Autodesk Inventor part; units mm, degrees
ref_plane "YZ Plane" through (0, 0, 0) normal (1, 0, 0) x (0, 1, 0)
sketch "Sketch1" plane through (0, 0, 0) normal (0, 0, 1) x (1, 0, 0)
  line L0 (0, 0) -> (1.778, 0)
  line L1 (1.778, 0) -> (1.778, 5.08)
  line L2 (1.778, 5.08) -> (0, 5.08)
  line L3 (0, 5.08) -> (0, 0)
  line L4 (1.778, 0) -> (11.049, 0)
  line L5 (11.049, 0) -> (11.049, 3.683)
  line L6 (11.049, 3.683) -> (1.778, 3.683)
  line L7 (1.778, 3.683) -> (1.778, 0)
  line L8 (8.509, 3.683) -> (6.985, 3.81)
  line L9 (6.985, 3.81) -> (6.985, 3.683)
  line L10 (6.985, 3.683) -> (5.461, 3.81)
  line L11 (5.461, 3.81) -> (5.461, 3.683)
  line L12 (5.461, 3.683) -> (3.937, 3.81)
  line L13 (3.937, 3.81) -> (3.937, 3.683)
  line L14 (0, 0) -> (0, 3.1252)
  line L15 (0, 3.81) -> (0.889, 3.81) construction
  line L16 (0, 3.81) -> (0, 0)
  arc A0 (0, 3.81) -> (-9.906, 3.556) centre (0, -189.484) ccw
  line L17 (-9.906, 3.556) -> (-9.906, 3.81)
  line L18 (-9.906, 3.81) -> (-11.176, 3.81)
  line L19 (-11.176, 3.81) -> (-11.176, 0)
  line L20 (-11.176, 0) -> (0, 0)
  dimension "d0" = 1.778
  dimension "d1" = 10.16
  dimension "d2" = 9.271
  dimension "d3" = 7.366
  dimension "d4" = 7.62
  dimension "d5" = 2.54
  dimension "d6" = 1.524
  dimension "d7" = 7.62
  dimension "d8" = 7.62
  dimension "d9" = 11.176
  dimension "d10" = 7.112
  dimension "d11" = 1.27
revolve "Revolution1" add sketch "Sketch1" angle 360 about axis through (-11.176, 0, 0) along (1, 0, 0)
sketch "Sketch2" plane through (0, 0, 0) normal (0, 0, 1) x (1, 0, 0)
  line L0 (-11.176, 0.508) -> (-6.096, 0.508)
  line L1 (-6.096, 0.508) -> (-6.096, -0.508)
  line L2 (-6.096, -0.508) -> (-11.176, -0.508)
  line L3 (-11.176, -0.508) -> (-11.176, 0.508)
  line L4 (-11.176, -3.81) -> (-11.176, 3.81) construction
  point P0 (0, 0)
  point P1 (-11.176, 0)
  dimension "d13" = 1.016
  dimension "d14" = 5.08
extrude "Extrusion1" cut sketch "Sketch2" along normal through all both and the other way through all
hole "Hole1" at (-11.176, 0, 0) direction (1, 0, 0) diameter 4.7625 depth 11.1125 counterbore diameter 6.35 counterbore depth 6.35
hole "Hole2" at (11.049, 0, 0) direction (-1, 0, 0) diameter 4.7625 depth 9.525 counterbore diameter 6.35 counterbore depth 1.27
sketch "Sketch3" plane through (1.778, 0, 0) normal (1, 0, 0) x (0, 0, -1)
  circle A0 centre (0, 0) radius 5.08
  circle A1 centre (0, 0) radius 5.08
  circle A2 centre (0, 0) radius 3.683
  circle A3 centre (0, 0) radius 3.81
  circle A4 centre (0, 0) radius 3.81
  circle A5 centre (0, 0) radius 3.81
  circle A6 centre (0, 0) radius 3.683
extrude "Extrusion2" cut sketch "Sketch3" against normal blind 1.778 contours A0
extrude "Extrusion3" add sketch "Sketch3" along normal blind 2.159 contours A3
sketch "Sketch4" plane through (11.049, 0, 0) normal (1, 0, 0) x (0, 0, -1)
  circle A0 centre (0, 0) radius 3.683
  circle A1 centre (0, 0) radius 3.175
extrude "Extrusion4" add sketch "Sketch4" along normal blind 29.21
mirror "Mirror1" about plane through (40.259, 0, 0) normal (1, 0, 0) of "Revolution1", "Extrusion1", "Hole1", "Hole2", "Extrusion2", "Extrusion3", "Extrusion4"
ref_plane "Work Plane2" through (25.4, 0, 0) normal (-1, 0, 0) x (0, 0, 1)
sketch "Sketch7" plane through (25.4, 0, 0) normal (-1, 0, 0) x (0, 0, 1)
  circle A0 centre (0, 0) radius 5.715
  line L0 (0, 8.001) -> (0, -8.001)
  line L1 (0.635, 6.477) -> (-0.635, 6.477)
  line L2 (-0.635, 6.477) -> (-0.635, 5.6796)
  line L3 (-0.635, 5.461) -> (0, 5.461)
  line L4 (0.635, 5.6796) -> (0.635, 6.477)
  dimension "d43" = 11.43
  dimension "d44" = 0.635
  dimension "d45" = 0.635
  dimension "d46" = 0.254
  dimension "d47" = 0.762
extrude "Extrusion5" add sketch "Sketch7" along normal mid plane 1.27 contours A0 L0 | A0 L0
extrude "Extrusion6" add sketch "Sketch7" along normal mid plane 1.27 contours A0 L0 L1 L4 | A0 L2 L1 L0
pattern_circular "Circular Pattern1" count 13 over 360 about axis through (25.4, 0, 0) along (-1, 0, 0) of "Extrusion6"
ref_plane "Work Plane3" through (34.544, 0, 0) normal (-1, 0, 0) x (0, 0, 1)
sketch "Sketch8" plane through (-11.176, 0, 0) normal (-1, 0, 0) x (0, 0, 1)
  circle A0 centre (0, 0) radius 2.3813
  circle A1 centre (0, 0) radius 16.574
  point P0 (0, 0)
extrude "Extrusion7" cut sketch "Sketch8" against normal blind 45.72 contours A0 | A1
sketch "Sketch9" plane through (34.544, 0, 0) normal (-1, 0, 0) x (0, 0, 1)
  circle A0 centre (0, 0) radius 3.175
  circle A1 centre (0, 0) radius 3.175
  circle A2 centre (0, 0) radius 2.667
  circle A3 centre (0, 0) radius 3.683
  circle A4 centre (0, 0) radius 3.683
  dimension "d58" = 0.508
extrude "Extrusion8" add sketch "Sketch9" against normal blind 10.16 contours A0
extrude "Extrusion9" cut sketch "Sketch9" against normal blind 5.08 contours A3
sketch "Sketch10" plane through (0, 0, 0) normal (0, 0, 1) x (1, 0, 0)
  line L0 (34.544, -2.667) -> (44.704, -2.667)
  line L1 (34.544, -3.175) -> (39.624, -3.175)
  line L2 (-18.3388, 0) -> (110.0328, 0)
  line L3 (34.544, 3.175) -> (39.624, 3.175)
  line L4 (39.624, 3.175) -> (39.624, 2.667)
  line L5 (39.624, 2.667) -> (34.544, 2.667)
  line L6 (34.544, 2.667) -> (34.544, 3.175)
  line L7 (34.544, -3.175) -> (39.624, -3.175)
  line L8 (39.624, -3.175) -> (39.624, -2.667)
  line L9 (39.624, -2.667) -> (34.544, -2.667)
  line L10 (34.544, -2.667) -> (34.544, -3.175)
  point P0 (0, 0)
  dimension "d63" = 5.08
revolve "Revolution2" cut sketch "Sketch10" angle 65 about axis through (0, 0, 0) along (1, 0, 0)
sketch "Sketch11" plane through (0, 0, 0) normal (0, 0, 1) x (1, 0, 0)
  line L0 (39.624, 3.175) -> (37.084, 3.175)
  line L1 (37.084, 3.175) -> (37.084, 2.667)
  line L2 (37.084, 2.667) -> (39.624, 2.667)
  line L3 (39.624, 2.667) -> (39.624, 3.175)
  line L4 (34.544, 1.1271) -> (39.624, 1.1271)
  line L5 (-18.3388, 0) -> (110.0328, 0)
  line L6 (39.624, -3.175) -> (37.084, -3.175)
  line L7 (37.084, -3.175) -> (37.084, -2.667)
  line L8 (37.084, -2.667) -> (39.624, -2.667)
  line L9 (39.624, -2.667) -> (39.624, -3.175)
  point P0 (0, 0)
  dimension "d65" = 2.54
revolve "Revolution3" cut sketch "Sketch11" angle 30 about axis through (0, 0, 0) along (-1, 0, 0)
equation "\"d8\" = d7"
properties part number "Motor Axle"
Geometry check sheet. Reference: the model listing, model coordinates, mm. A direction names the side the tool comes from. Coordinates: 2 decimals unless noted, no trailing zeros. Order: outer loops, then holes, each group sorted by start corner. A loop starts at its lowest first (then second) coordinate and runs counter-clockwise, first axis right, second up. Notation, with made-up numbers: (-6, 1.25) - (45, 1.25) arc R33 cw to (45, 34.25) - close; hole circle Ø1 at (38, 51). An arc over 180 degrees is marked (long way). Answer in a Markdown table with one row per item. Add a question column.
1) Cross-section at C-C, the plane x = 80. Record the cut outline in (y, z).
2) Material ranges on line 1 along Y through (x, z) = (65, 0) (3 decimals); line 2 along Y through (x, z) = (75.5, 0); line 3 along Z through (x, y) = (40.25, 0), recorded low to high. Write a range as [from, to].
3) Cross-section at B-B, the plane x = 70. Record the cut outline in (y, z) (3 decimals).
4) Set-up check for faces 1 (the cylindrical face through (37.048, -1.743, 2.654)), 2 (the cylindrical face through (88.47, 0.95, 3.03)), 3 (the flat face through (78.994, 0, 0)), 4 (the cylindrical face through (37.048, 1.743, -2.654)), 5 (the conical face through (73.967, 3.436, -1.424)): record each of +Z, -Z, +X, -X, +Y, -Y from which the full face is reachable in a straight line by a thin tool's end or side.
5) Release check for a two-part mould opening along Z. For faces 6 (the cylindrical face through (57.9, -3.1, 0.69)), 7 (the cylindrical face through (91.07, -3.81, 0.08)), 8 (the flat face through (91.694, -3.3, -0.5)) record: +Z half, -Z half, draft (parallel to the pull), parting line (faces both ways), or undercut.
6) Gauge pin test, flat ends, axial feed: P1, Ø2.5, axis at y = 0, z = 0, coming from the +X side; P2, Ø1, axis at x = 83, z = 2.5, coming from the -Y side; P3, Ø3, axis at x = 52, z = -2.5, coming from the +Y side. Record the tip position at first contact, or that the pin passes through.
Check result:
| question | item | result |
|---|---|---|
| 1 | outline | circle Ø7.62 at (0, 0) |
| 2 | line 1 | y = [-3.683, -3.175], [3.175, 3.683] |
| 2 | line 2 | y = [-3.72, -2.38], [2.38, 3.72] |
| 2 | line 3 | z = [-3.68, -2.67], [2.67, 3.68] |
| 3 | outline | circle Ø7.366 at (0, 0); hole circle Ø6.35 at (0, 0) |
| 4 | face 1 | +Z, -X |
| 4 | face 2 | +X |
| 4 | face 3 | -X |
| 4 | face 4 | -Z, -X |
| 4 | face 5 | none |
| 5 | face 6 | undercut |
| 5 | face 7 | parting line |
| 5 | face 8 | draft |
| 6 | P1 | stops at x = 80.58 |
| 6 | P2 | stops at y = -3.22 |
| 6 | P3 | stops at y = 3.54 |
